Check sheet for the drawn part. Datum: minimum x, y, z corner. Units: mm. Give positions to 0.01 mm unless a question says otherwise; leave off trailing zeros. Loops run counter-clockwise (first coordinate to the right, second up) from the corner with the lowest first, then second, coordinate; pieces in that order, holes last. Notation, with made-up numbers: (67, -20.5) - (82, -20.5) arc R29 ccw to (82, 5.5) - close; hole circle Ø9 at (15.25, 38.5). An arc over 180 degrees is marked (long way). One line per item, written item: value. Start each with the question number.
1. Scan lines: L1, parallel to Z at x = 121, y = 0.75; L2, parallel to X at y = 2.45, z = 34 (1 decimal); L3, parallel to Z at x = 30, y = 1.2. Record each from-to range of solid material in increasing order. Write a range as [from, to].
2. Sectioned sample at A-A (x = 115). Record the cut outline in (y, z), plus the area to 3 significant figures.
3. Sectioned sample at D-D (x = 99.5). Record the cut outline in (y, z), plus the area to 3 significant figures.
4. Sectioned sample at B-B (z = 31.75). Record the cut outline in (x, y), plus the area to 3 significant figures.
5. Sectioned sample at C-C (y = 1.2). Count the separate pieces of the cut face and the enclosed holes in it, plus the area to 3 significant figures.
6. Gauge pin test, flat ends, axial feed: pin 1 (1.5 mm diameter, centred on x = 2, y = 1.5, fed in from +Z); pin 2 (0.9 mm diameter, centred on y = 1.5, z = 62.5, fed in from +X). Record the tip position at first contact, or that the pin passes through.
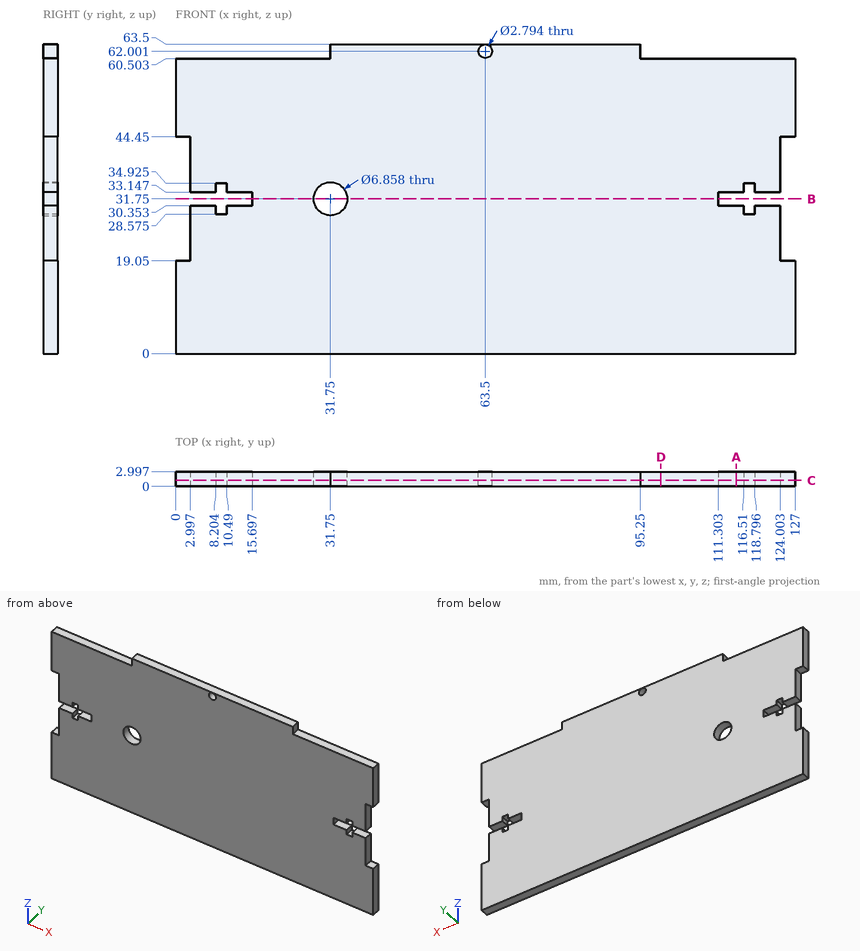
Results are:
1. L1: z = [0, 30.35], [33.15, 60.5]
1. L2: x = [3, 8.2], [10.5, 29.2], [34.3, 116.5], [118.8, 124]
1. L3: z = [0, 28.8], [34.7, 60.5]
2. outline: (0, 0) - (3, 0) - (3, 30.35) - (0, 30.35) - close; (0, 33.15) - (3, 33.15) - (3, 60.5) - (0, 60.5) - close
2. area: 173 mm^2
3. outline: (0, 0) - (3, 0) - (3, 60.5) - (0, 60.5) - close
3. area: 181 mm^2
4. outline: (15.7, 0) - (28.32, 0) - (28.32, 3) - (15.7, 3) - close; (35.18, 0) - (111.3, 0) - (111.3, 3) - (35.18, 3) - close
4. area: 266 mm^2
5. separate pieces: 1
5. enclosed holes: 2
5. area: 7,590 mm^2
6. pin 1: stops at z = 60.5
6. pin 2: stops at x = 95.25
